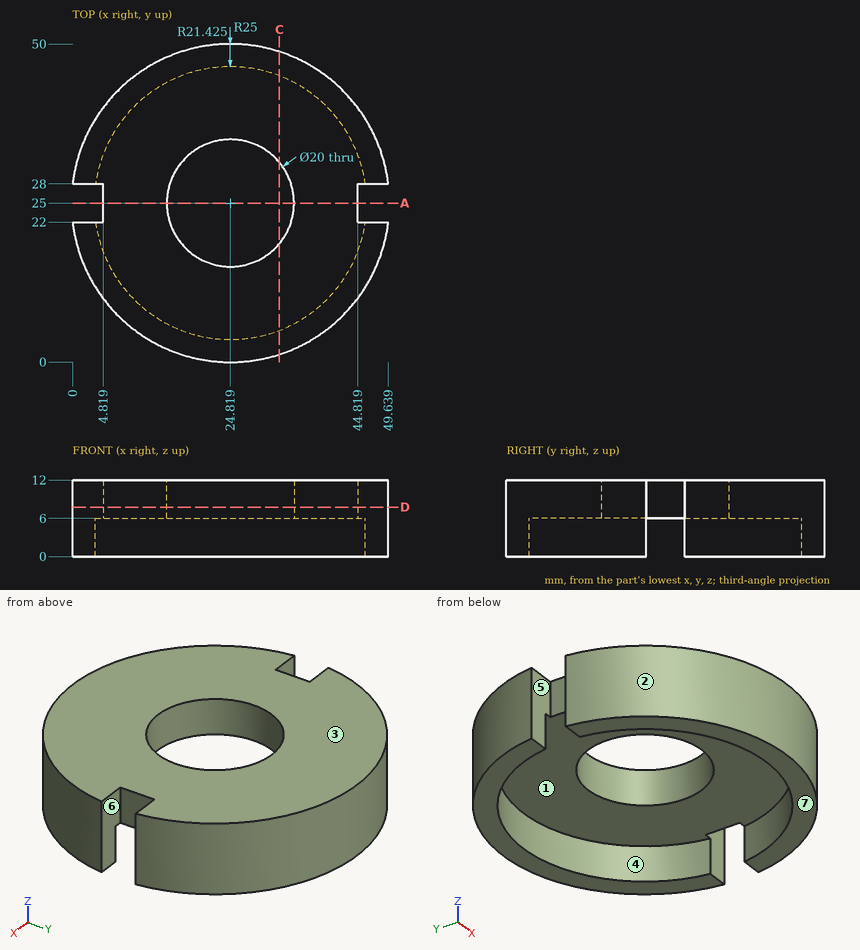
Geometry check sheet. Reference: drawing and pictorial views, mm from the part's lowest x, y, z. A direction names the side the tool comes from. Give positions to 0.01 mm unless a question says otherwise; leave off trailing zeros. Order: outer loops, then holes, each group sorted by start corner. A loop starts at its lowest first (then second) coordinate and runs counter-clockwise, first axis right, second up. Notation, with made-up numbers: (-37.75, 75.25) - (-27.75, 75.25) arc R24 cw to (-27.75, 106.25) - close; hole circle Ø8 at (8.5, 29.25). An arc over 180 degrees is marked (long way). Use one line per item in the form item = value.
1) Access from +Z, -Z, +X, -X, +Y, -Y to the whole of each face (thin tool, end or side, straight path). Record for the marked faces 4, 5, 6 and 7.
Working result:
face_4 = -Z
face_5 = +Z, -Z, -X
face_6 = +Z, -Z, +X
face_7 = -Z, +X, -X, +Y, -Y
2) Sectioned sample at D-D (z = 7.75). Record the boundary of the cut face in (x, y), and give its area (3 significant figures).
Working result:
outline = (0, 22) arc R25 ccw to (49.64, 22) - (44.82, 22) - (44.82, 28) - (49.64, 28) arc R25 ccw to (0, 28) - (4.82, 28) - (4.82, 22) - close; hole circle Ø20 at (24.82, 25)
area = 1,590 mm^2
3) Depth check by flat-ended pin: pin 1 Ø6 at (y, z) = (33, 5.5) entering from +X; pin 2 Ø3 at (y, z) = (25.5, 7.5) entering from -X; pin 3 Ø1.4 at (x, z) = (46.5, 7.5) entering from -Y (1 decimal). Enter the tip coordinate at first touch or a pass-through.
Working result:
pin_1 = 49.31
pin_2 = 4.82
pin_3 = 11.4
4) Draft check along X on the marked faces 1, 2 and 3. Enter one of: released by +X, released by -X, zero draft, split by the parting line, or undercut.
Working result:
face_1 = undercut
face_2 = split by the parting line
face_3 = zero draft
5) Sectioned sample at A-A (y = 25). Record the boundary of the cut face in (x, z).
Working result:
outline = (4.82, 6) - (14.82, 6) - (14.82, 12) - (4.82, 12) - close; (34.82, 6) - (44.82, 6) - (44.82, 12) - (34.82, 12) - close
6) Sectioned sample at C-C (x = 32.5). Record the boundary of the cut face in (y, z), and give its area (3 significant figures).
Working result:
outline = (1.21, 0) - (5, 0) - (5, 6) - (18.6, 6) - (18.6, 12) - (1.21, 12) - close; (31.4, 6) - (45, 6) - (45, 0) - (48.79, 0) - (48.79, 12) - (31.4, 12) - close
area = 254 mm^2
7) Material ranges on probe 1 along X at (y, z) = (25.5, 10); probe 2 along Z at (x, y) = (24.5, 43.5); probe 3 along X at (y, z) = (34, 7) (1 decimal), recorded low to high. Write a range as from..to.
Working result:
probe_1 = 4.82..14.83, 34.81..44.82
probe_2 = 6..12
probe_3 = 1.5..20.5, 29.2..48.1
